Read the model definition and answer for the solid it produces. Units are mm, in the model's axes. Face numbers are marked on the shaded views. A direction names the side the tool comes from. Give positions to 0.01 mm unless a question says otherwise; leave off trailing zeros. Loops run counter-clockwise (first coordinate to the right, second up) from the corner with the lowest first, then second, coordinate; pieces in that order, holes last. Notation, with made-up numbers: (-20.75, 32.25) - (26.25, 32.25) arc R13 cw to (26.25, 46.25) - close; hole circle Ø3 at (28.5, 59). An arc over 180 degrees is marked (long way). Put each result on its own line as item: value. Start each with the question number.
1. A cutting plane is placed at C-C, the plane y = 61. Determine the outline of the cut face in (x, z).
2. For the marked faces 4, 5 and 6, determine the directions among +Z, -Z, +X, -X, +Y, -Y from which every point of the face is accessible in a straight line to the end or side of a thin tool.
3. For a pull along Y with two mould halves and no side action, classify the marked faces 1, 2 and 3 as released by +Y, released by -Y, zero draft, split by the parting line, or undercut.
4. A cutting plane is placed at B-B, the plane z = 13.5. Determine the outline of the cut face in (x, y).
5. Given pin 1 Ø6 at (y, z) = (-16.5, 34.5) entering from +X; pin 2 Ø15 at (y, z) = (47.5, 34.5) entering from -X, each flat-ended and moving along its own axis, determine where each tip first touches the part or whether it passes through.
6. Consider L1, parallel to Y at x = 65.5, z = 23; L2, parallel to Y at x = -22.5, z = 29; L3, parallel to X at y = 74.5, z = 27. Determine where each line is inside the solid, lowest interval first. Write a range as from..to.
7. A cutting plane is placed at D-D, the plane y = 118. Determine the outline of the cut face in (x, z).
8. A cutting plane is placed at A-A, the plane x = 106. Determine the outline of the cut face in (y, z).
```python
from build123d import *

# Parameters (mm, degrees)
EXTRUDE_DEPTH = 50


with BuildPart() as part:
    # Sketch → Extrude (new body)
    with BuildSketch(Plane.XY):
        with BuildLine():
            Line((5.75, -112.5), (5.75, 112.5))
            ThreePointArc((32.75, 139.5), (13.658117, 131.591883), (5.75, 112.5))
            Line((32.75, 139.5), (150, 139.5))
            Line((150, 139.5), (150, 160))
            Line((150, 160), (-150, 160))
            Line((-150, 160), (-150, 139.5))
            Line((-150, 139.5), (-32.75, 139.5))
            ThreePointArc((-5.75, 112.5), (-13.658117, 131.591883), (-32.75, 139.5))
            Line((-5.75, 112.5), (-5.75, -112.5))
            ThreePointArc((-32.75, -139.5), (-13.658117, -131.591883), (-5.75, -112.5))
            Line((-32.75, -139.5), (-150, -139.5))
            Line((-150, -139.5), (-150, -160))
            Line((-150, -160), (150, -160))
            Line((150, -160), (150, -139.5))
            Line((150, -139.5), (32.75, -139.5))
            ThreePointArc((5.75, -112.5), (13.658117, -131.591883), (32.75, -139.5))
        make_face()
    extrude(amount=EXTRUDE_DEPTH)


solid = part.part
```
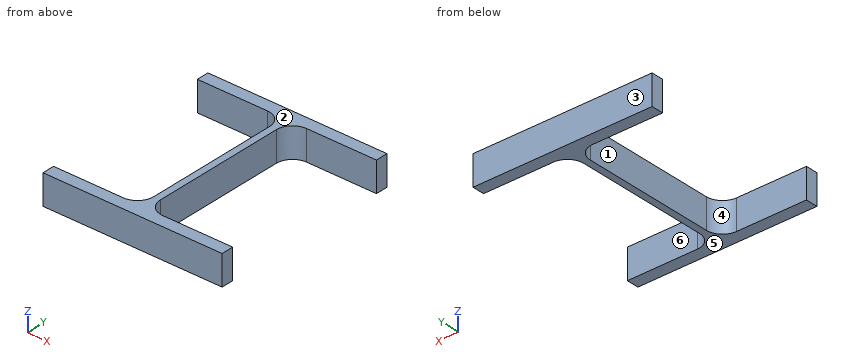
Return value:
1. outline: (-5.75, 0) - (5.75, 0) - (5.75, 50) - (-5.75, 50) - close
2. face 4: +Z, -Z, -X
2. face 5: -Z, +X, -X, +Y, -Y
2. face 6: +Z, -Z, +X
3. face 1: undercut
3. face 2: zero draft
3. face 3: released by +Y
4. outline: (-150, -160) - (150, -160) - (150, -139.5) - (32.75, -139.5) arc R27 cw to (5.75, -112.5) - (5.75, 112.5) arc R27 cw to (32.75, 139.5) - (150, 139.5) - (150, 160) - (-150, 160) - (-150, 139.5) - (-32.75, 139.5) arc R27 cw to (-5.75, 112.5) - (-5.75, -112.5) arc R27 cw to (-32.75, -139.5) - (-150, -139.5) - close
5. pin 1: stops at x = 5.75
5. pin 2: stops at x = -5.75
6. L1: y = -160..-139.5, 139.5..160
6. L2: y = -160..-137.48, 137.48..160
6. L3: x = -5.75..5.75
7. outline: (-6.32, 0) - (6.32, 0) - (6.32, 50) - (-6.32, 50) - close
8. outline: (-160, 0) - (-139.5, 0) - (-139.5, 50) - (-160, 50) - close; (139.5, 0) - (160, 0) - (160, 50) - (139.5, 50) - close
